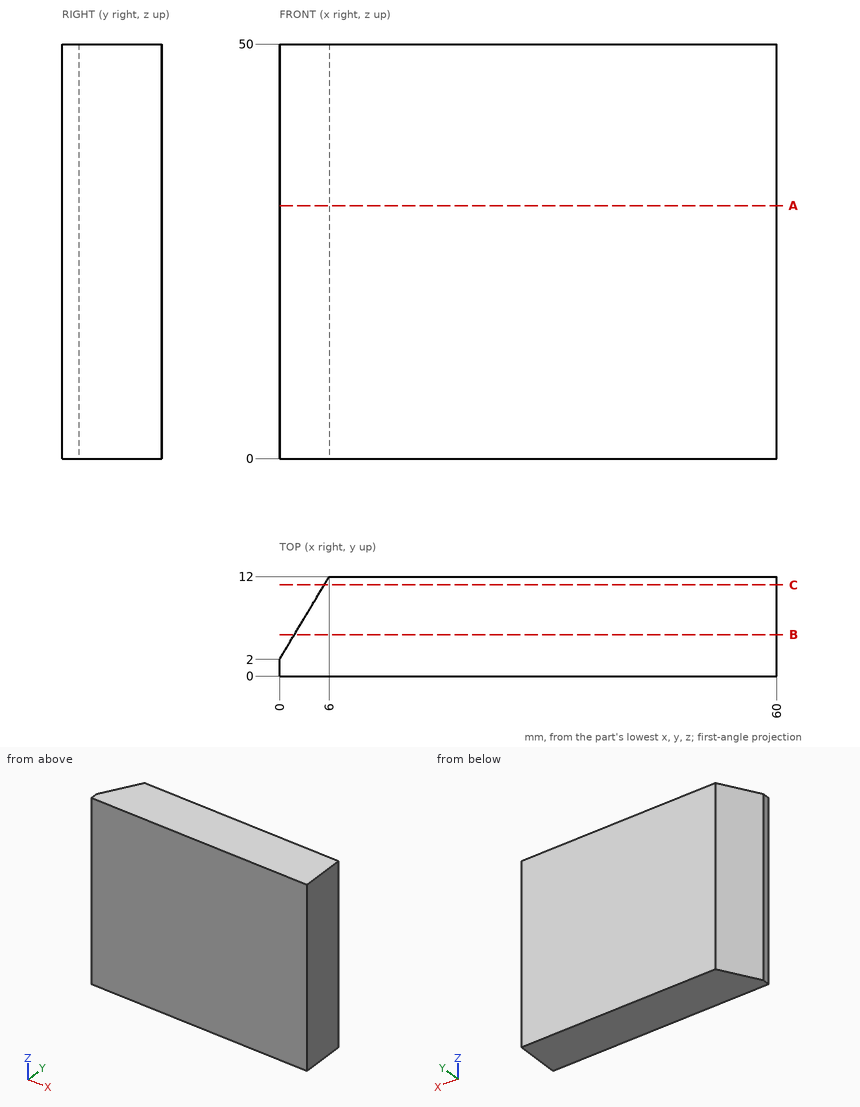
Here's the drawing with two shaded views (mm, measured from the low corner). I have some questions. Coordinates: 2 decimals unless noted, no trailing zeros. Order: outer loops, then holes, each group sorted by start corner. A loop starts at its lowest first (then second) coordinate and runs counter-clockwise, first axis right, second up.
Q1. Suppose I cut it at C-C on y = 11. Please give me the cut outline in (x, z), and give its area (3 significant figures).
Q2. Suppose I cut it at B-B on y = 5. Please give me the cut outline in (x, z), and give its area (3 significant figures).
Q3. Please list where these lines run through material, in increasing order: L1, parallel to X at y = 5.25, z = 33.5; L2, parallel to X at y = 7, z = 8; L3, parallel to Y at x = 3, z = 2.
Q4. Will these pins go through, and if not, where does the flat tip stop? pin 1 (4 mm diameter, centred on y = 7, z = 19, fed in from -X); pin 2 (6 mm diameter, centred on y = 10.5, z = 25.5, fed in from -X).
Q5. Suppose I cut it at A-A on z = 30.5. Please give me the cut outline in (x, y), and give its area (3 significant figures).
Answer:
1. outline: (5.4, 0) - (60, 0) - (60, 50) - (5.4, 50) - close
1. area: 2,730 mm2
2. outline: (1.8, 0) - (60, 0) - (60, 50) - (1.8, 50) - close
2. area: 2,910 mm2
3. L1: x = 1.95 to 60
3. L2: x = 3 to 60
3. L3: y = 0 to 7
4. pin 1: stops at x = 1.8
4. pin 2: stops at x = 3.3
5. outline: (0, 0) - (60, 0) - (60, 12) - (6, 12) - (0, 2) - close
5. area: 690 mm2
